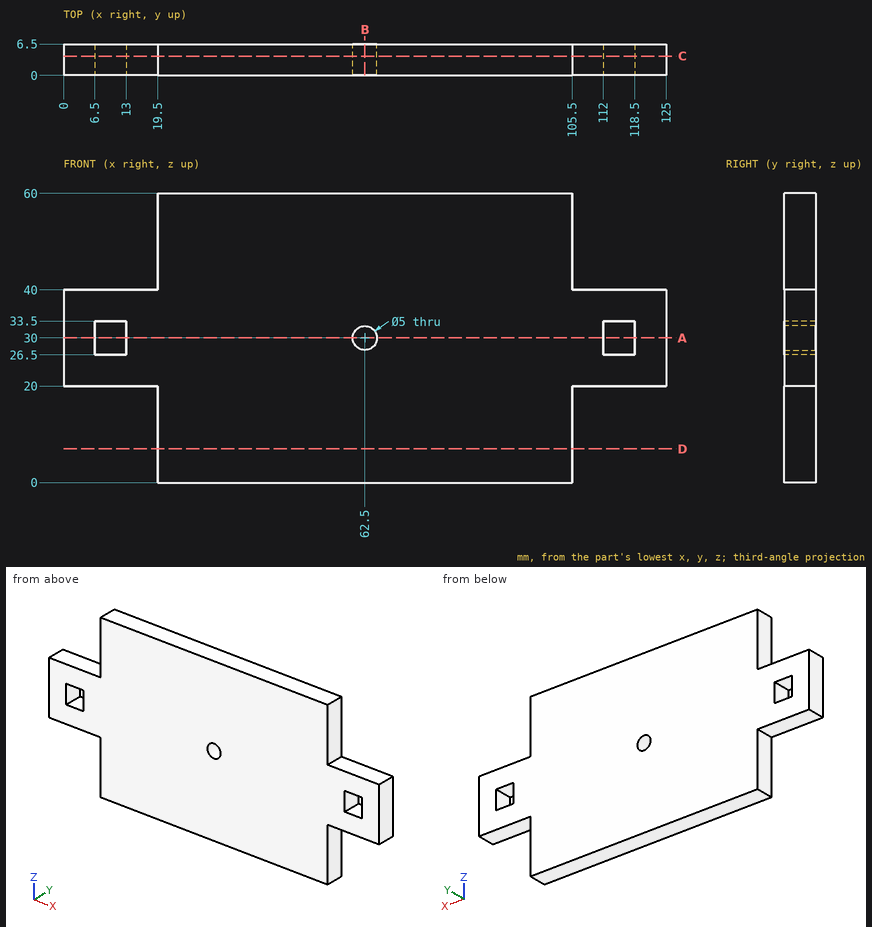
Geometry: see drawing. Coordinates: mm, zero at the bounding-box minimum. Coordinates: 2 decimals unless noted, no trailing zeros. Write each loop counter-clockwise with the first axis right and the second up, starting at its lowest first coordinate (ties: lowest second). Pieces come first, ordered by that corner, then holes.
1) Section D-D on z = 7. Output: boundary loops of the cut face in (x, y), and give its area (3 significant figures).
2) Pin query (flat end, axial travel): pin 1 Ø3 at (x, z) = (92.5, 20) entering from -Y; pin 2 Ø1 at (y, z) = (4.5, 48.5) entering from -X; pin 3 Ø3 at (x, y) = (120, 2.5) entering from +Z; pin 4 Ø3 at (y, z) = (3.5, 13.5) entering from +X. Return the tip coordinate at first contact, or that it passes through.
3) Section A-A on z = 30. Output: boundary loops of the cut face in (x, y).
4) Section C-C on y = 4. Output: boundary loops of the cut face in (x, z), and give its area (3 significant figures).
5) Material intervals for line 1 along X through (y, z) = (2.5, 30); line 2 along Z through (x, y) = (117.5, 4); line 3 along X through (y, z) = (2.75, 8.5), sorted ascending.
6) Section B-B on x = 62.5. Output: boundary loops of the cut face in (y, z).
Check result:
1. outline: (19.5, 0) - (105.5, 0) - (105.5, 6.5) - (19.5, 6.5) - close
1. area: 559 mm2
2. pin 1: stops at y = 0
2. pin 2: stops at x = 19.5
2. pin 3: stops at z = 40
2. pin 4: stops at x = 105.5
3. outline: (0, 0) - (6.5, 0) - (6.5, 6.5) - (0, 6.5) - close; (13, 0) - (60, 0) - (60, 6.5) - (13, 6.5) - close; (65, 0) - (112, 0) - (112, 6.5) - (65, 6.5) - close; (118.5, 0) - (125, 0) - (125, 6.5) - (118.5, 6.5) - close
4. outline: (0, 20) - (19.5, 20) - (19.5, 0) - (105.5, 0) - (105.5, 20) - (125, 20) - (125, 40) - (105.5, 40) - (105.5, 60) - (19.5, 60) - (19.5, 40) - (0, 40) - close; hole (6.5, 26.5) - (13, 26.5) - (13, 33.5) - (6.5, 33.5) - close; hole circle Ø5 at (62.5, 30); hole (112, 26.5) - (118.5, 26.5) - (118.5, 33.5) - (112, 33.5) - close
4. area: 5,830 mm2
5. line 1: x = 0 to 6.5, 13 to 60, 65 to 112, 118.5 to 125
5. line 2: z = 20 to 26.5, 33.5 to 40
5. line 3: x = 19.5 to 105.5
6. outline: (0, 0) - (6.5, 0) - (6.5, 27.5) - (0, 27.5) - close; (0, 32.5) - (6.5, 32.5) - (6.5, 60) - (0, 60) - close
